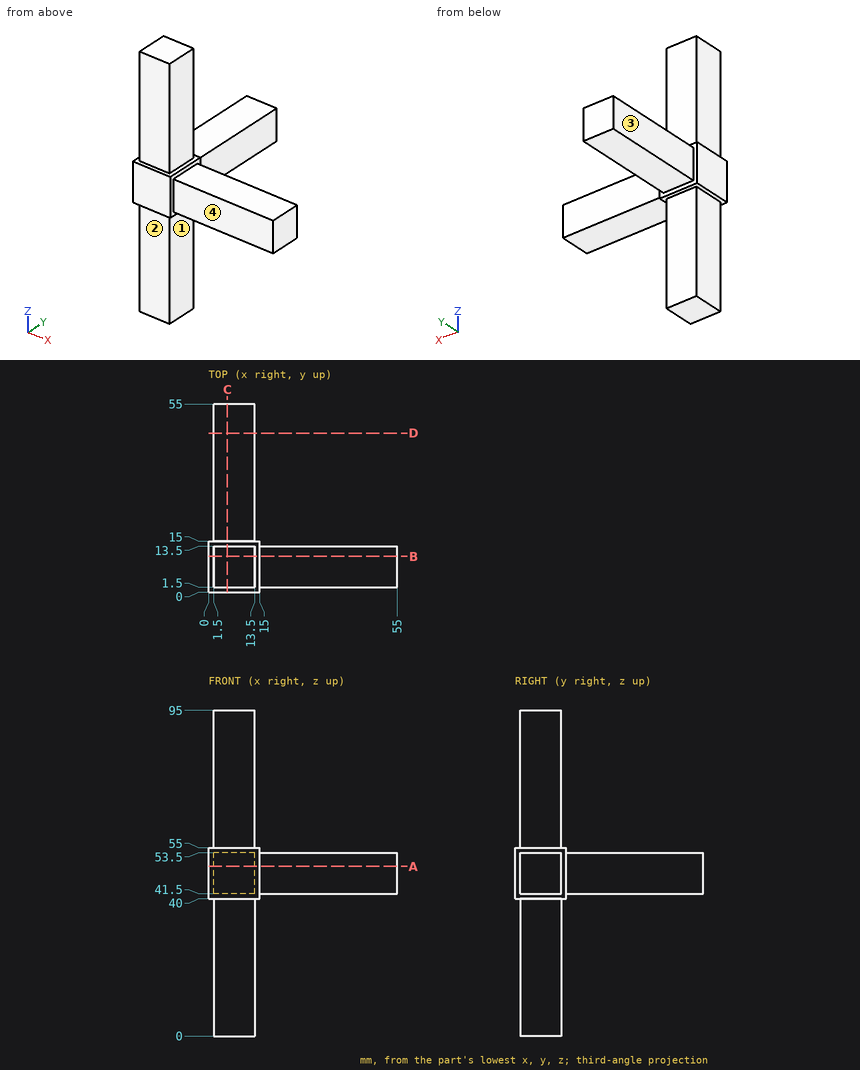
Verification items for this drawing (mm, ordinates from the low corner). A direction names the side the tool comes from. Coordinates: 2 decimals unless noted, no trailing zeros. Write each loop counter-clockwise with the first axis right and the second up, starting at its lowest first coordinate (ties: lowest second). Pieces come first, ordered by that corner, then holes. Notation, with made-up numbers: (-18, 82) - (-10, 82) arc R14 ccw to (-10, 95) - close; hole circle Ø7 at (20, 84). An arc over 180 degrees is marked (long way). One line per question, with ' | ' between items.
Item 1: Sectioned sample at B-B on y = 10.5. Record the boundary of the cut face in (x, z), plus the area to 4 significant figures.
Determined:
outline: (0, 40) - (1.5, 40) - (1.5, 0) - (13.5, 0) - (13.5, 40) - (15, 40) - (15, 41.5) - (55, 41.5) - (55, 53.5) - (15, 53.5) - (15, 55) - (13.5, 55) - (13.5, 95) - (1.5, 95) - (1.5, 55) - (0, 55) - close | area: 1,665 mm2
Item 2: Gauge pin test, flat ends, axial feed: P1, Ø12, axis at x = 5, y = 8, coming from the -Z side; P2, Ø9.5, axis at x = 7, z = 72, coming from the +Y side; P3, Ø10, axis at x = 14.5, y = 22, coming from the +Z side; P4, Ø3.5, axis at x = 28.5, y = 10, coming from the -Z side. Record the tip position at first contact, or that the pin passes through.
Determined:
P1: stops at z = 0 | P2: stops at y = 13.5 | P3: stops at z = 53.5 | P4: stops at z = 41.5
Item 3: Thickness scan on line 1 (X direction, y = 7, z = 36); line 2 (Z direction, x = 32, y = 12). Record the ranges inside material, lowest first. Write a range as [from, to].
Determined:
line 1: x = [1.5, 13.5] | line 2: z = [41.5, 53.5]
Item 4: Access from +Z, -Z, +X, -X, +Y, -Y to the whole of each face (thin tool, end or side, straight path). Record for the marked faces 1, 2, 3 and 4.
Determined:
face 1: -Z, +X, +Y, -Y | face 2: -Z, +X, -X, -Y | face 3: +Z, -Z, -X, +Y | face 4: +Z, -Z, +X, -Y
Item 5: Sectioned sample at A-A on z = 49.5. Record the boundary of the cut face in (x, y), plus the area to 4 significant figures.
Determined:
outline: (0, 0) - (15, 0) - (15, 1.5) - (55, 1.5) - (55, 13.5) - (15, 13.5) - (15, 15) - (13.5, 15) - (13.5, 55) - (1.5, 55) - (1.5, 15) - (0, 15) - close | area: 1,185 mm2
Item 6: Sectioned sample at D-D on y = 46.5. Record the boundary of the cut face in (x, z).
Determined:
outline: (1.5, 41.5) - (13.5, 41.5) - (13.5, 53.5) - (1.5, 53.5) - close
